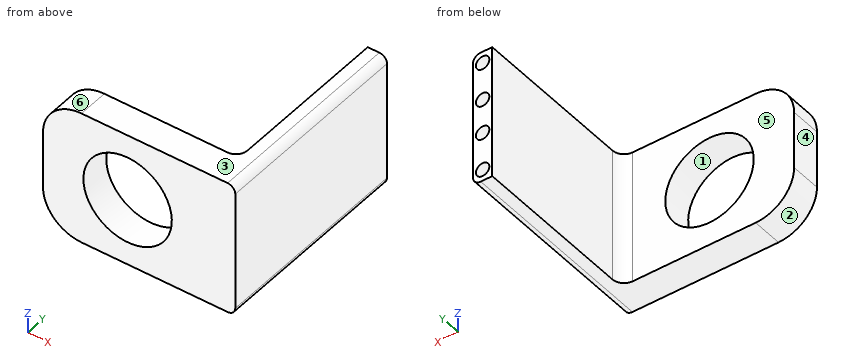
from build123d import *

# Parameters (mm, degrees)
SKETCH1_W           = 50
SKETCH1_H           = 35
SKETCH1_R           = 11.5
BOSS_EXTRUDE1_DEPTH = 8
SKETCH2_W           = 5
SKETCH2_H           = 35
BOSS_EXTRUDE2_DEPTH = 45
FILLET2_R           = 3
SKETCH5_R           = 1.75
CUT_EXTRUDE2_DEPTH  = 10
FILLET3_R           = 10
FILLET4_R           = 2


with BuildPart() as part:
    # Sketch1 → Boss-Extrude1 (new body)
    with BuildSketch(Plane(origin=(0, 0, 0), x_dir=(1, 0, 0), z_dir=(0, 1, 0))):
        with Locations((3, 0)):
            Rectangle(SKETCH1_W, SKETCH1_H)
        with Locations(Location((0, 0, 0), (0, 0, 270))):
            Circle(SKETCH1_R, mode=Mode.SUBTRACT)
    extrude(amount=BOSS_EXTRUDE1_DEPTH)

    # Sketch2 → Boss-Extrude2 (add)
    with BuildSketch(Plane(origin=(0, 8, 0), x_dir=(1, 0, 0), z_dir=(0, 1, 0))):
        with Locations((25.5, 0)):
            Rectangle(SKETCH2_W, SKETCH2_H)
    extrude(amount=BOSS_EXTRUDE2_DEPTH)

    # Fillet2
    fillet2_edges = [part.edges().sort_by_distance(p)[0] for p in [
        (23, 8, 0),
    ]]
    fillet(fillet2_edges, radius=FILLET2_R)

    # Sketch5 → Cut-Extrude2 (cut)
    with BuildSketch(Plane(origin=(0, 53, 0), x_dir=(1, 0, 0), z_dir=(0, 1, 0))):
        with Locations(Location((25.5, 14.5, 0), (0, 0, 270))):
            Circle(SKETCH5_R)
        with Locations(Location((25.5, -14.5, 0), (0, 0, 270))):
            Circle(SKETCH5_R)
        with Locations(Location((25.5, 4.5, 0), (0, 0, 270))):
            Circle(SKETCH5_R)
        with Locations(Location((25.5, -4.5, 0), (0, 0, 270))):
            Circle(SKETCH5_R)
    extrude(amount=-CUT_EXTRUDE2_DEPTH, mode=Mode.SUBTRACT)

    # Fillet3
    fillet3_edges = [part.edges().sort_by_distance(p)[0] for p in [
        (-22, 4, 17.5),
        (-22, 4, -17.5),
    ]]
    fillet(fillet3_edges, radius=FILLET3_R)

    # Fillet4
    fillet4_edges = [part.edges().sort_by_distance(p)[0] for p in [
        (28, 26.5, 17.5),
        (28, 26.5, -17.5),
    ]]
    fillet(fillet4_edges, radius=FILLET4_R)


solid = part.part
Verification items for the finished model (mm, model axes). Face numbers are marked on the shaded views. A direction names the side the tool comes from. Give positions to 0.01 mm unless a question says otherwise; leave off trailing zeros. Write each loop counter-clockwise with the first axis right and the second up, starting at its lowest first coordinate (ties: lowest second). Pieces come first, ordered by that corner, then holes.
(1) Mould release check, pull along Z, two halves, no side actions. Record for the marked faces 1, 2, 3 and 4: +Z half, -Z half, draft (parallel to the pull), parting line (faces both ways), or undercut.
(2) Cross-section at A-A (x = 0). Enter the section's corners in (y, z), plus the area to 3 significant figures.
(3) Material ranges on line 1 (X direction, y = 49, z = -4.5); line 2 (X direction, y = 3.25, z = 0); line 3 (X direction, y = 44.5, z = 0.5), recorded low to high.
(4) Gauge pin test, flat ends, axial feed: pin 1 (3 mm diameter, centred on x = 25.5, z = 4.5, fed in from +Y); pin 2 (17.5 mm diameter, centred on x = 0.5, z = -3, fed in from +Y); pin 3 (18.5 mm diameter, centred on x = 0, z = 0, fed in from -Y). Record the tip position at first contact, or that the pin passes through.
(5) Cross-section at D-D (y = 27.5). Enter the section's corners in (x, z).
(6) Access from +Z, -Z, +X, -X, +Y, -Y to the whole of each face (thin tool, end or side, straight path). Record for the marked faces 5 and 6.
(7) Cross-section at C-C (y = 47). Enter the section's corners in (x, z).
(8) Cross-section at B-B (z = 0). Enter the section's corners in (x, y), plus the area to 3 significant figures.
Worked out:
1. face 1: undercut
1. face 2: -Z half
1. face 3: +Z half
1. face 4: draft
2. outline: (0, -17.5) - (8, -17.5) - (8, -11.5) - (0, -11.5) - close; (0, 11.5) - (8, 11.5) - (8, 17.5) - (0, 17.5) - close
2. area: 96.0 mm2
3. line 1: x = 23 to 23.75, 27.25 to 28
3. line 2: x = -22 to -11.5, 11.5 to 28
3. line 3: x = 23 to 28
4. pin 1: stops at y = 43
4. pin 2: stops at y = 8
4. pin 3: passes through
5. outline: (23, -17.5) - (26, -17.5) arc R2 ccw to (28, -15.5) - (28, 15.5) arc R2 ccw to (26, 17.5) - (23, 17.5) - close
6. face 5: +Z, -Z, -X, +Y
6. face 6: +Z, -X, +Y, -Y
7. outline: (23, -17.5) - (26, -17.5) arc R2 ccw to (28, -15.5) - (28, 15.5) arc R2 ccw to (26, 17.5) - (23, 17.5) - close; hole circle Ø3.5 at (25.5, -14.5); hole circle Ø3.5 at (25.5, -4.5); hole circle Ø3.5 at (25.5, 4.5); hole circle Ø3.5 at (25.5, 14.5)
8. outline: (-22, 0) - (-11.5, 0) - (-11.5, 8) - (-22, 8) - close; (11.5, 0) - (28, 0) - (28, 53) - (23, 53) - (23, 11) arc R3 cw to (20, 8) - (11.5, 8) - close
8. area: 443 mm2
